Source: CAD feature listing. Evaluate the final solid. Frame: model axes, mm. A direction names the side the tool comes from. Give positions to 0.01 mm unless a question says otherwise; leave off trailing zeros. Write each loop counter-clockwise with the first axis right and the second up, starting at its lowest first coordinate (ties: lowest second). Pieces come first, ordered by that corner, then holes.
```python
from build123d import *

# Parameters (mm, degrees)
SKETCH_1_R          = 2
EXTRUDE_1_DEPTH     = 4
FILLET_1_R          = 10
FILLET_2_R          = 2
SKETCH_8_R          = 3.300000000000001
EXTRUDE_3_DEPTH     = 5
CHAMFER_1_SIZE      = 5
SKETCH_9_R          = 3.300000000000001
CUT_EXTRUDE_3_DEPTH = 5
CHAMFER_2_SIZE      = 5
SKETCH_10_R         = 5.5
SKETCH_10_R_2       = 3.3000000000000003
EXTRUDE_4_DEPTH     = 4
SKETCH_11_R         = 3.3000000000000007
CUT_EXTRUDE_4_DEPTH = 4
FILLET_3_R          = 5
SKETCH_12_R         = 1.7999999999999998
SKETCH_12_R_2       = 1.800000000000001
SKETCH_12_R_3       = 1.7999999999999972
SKETCH_12_R_4       = 1.8000000000000007
CUT_EXTRUDE_5_DEPTH = 10


with BuildPart() as part:
    # ｽｹｯﾁ1 → ﾎﾞｽ - 押し出し1 (new body)
    # profile 1 of 5: a face of its own
    with BuildSketch(Plane.XY):
        with BuildLine():
            ThreePointArc((-27.5, 2.1540659228538024), (-27.33345237791561, 2.333452377915602), (-27.15406592285381, 2.49999999999999))
            Line((-27.154065922853814, 2.499999999999997), (-27.499999999999996, 2.499999999999997))
            Line((-27.499999999999996, 2.499999999999997), (-27.499999999999996, 2.154065922853802))
        make_face()
    # profile 2 of 5: a face of its own
    with BuildSketch(Plane.XY):
        with BuildLine():
            Line((-27.5, -2.500000000000003), (-27.154065922853817, -2.500000000000003))
            ThreePointArc((-27.154065922853817, -2.499999999999992), (-27.333452377915613, -2.3334523779156044), (-27.5, -2.1540659228538055))
            Line((-27.5, -2.1540659228538055), (-27.5, -2.500000000000003))
        make_face()
    # profile 3 of 5: a face of its own
    with BuildSketch(Plane.XY):
        with BuildLine():
            ThreePointArc((-20.10102051443362, 2.49999999999994), (-30.499999999999996, -2.39e-15), (-20.101020514433618, -2.4999999999999454))
            Line((-20.1010205144336, -2.500000000000002), (-22.84593407714621, -2.5000000000000027))
            ThreePointArc((-22.845934077146207, -2.5000000000000133), (-25.000000000000018, -3.3000000000000043), (-27.154065922853817, -2.499999999999992))
            Line((-27.154065922853817, -2.500000000000003), (-27.5, -2.500000000000003))
            Line((-27.5, -2.500000000000003), (-27.5, -2.1540659228538055))
            ThreePointArc((-27.5, -2.1540659228538055), (-28.3, -1.19e-15), (-27.5, 2.1540659228538024))
            Line((-27.499999999999996, 2.154065922853802), (-27.499999999999996, 2.499999999999997))
            Line((-27.499999999999996, 2.499999999999997), (-27.154065922853814, 2.499999999999997))
            ThreePointArc((-27.15406592285381, 2.49999999999999), (-25.000000000000014, 3.299999999999998), (-22.845934077146207, 2.500000000000007))
            Line((-22.84593407714621, 2.4999999999999982), (-20.1010205144336, 2.4999999999999987))
        make_face()
    # profile 4 of 5: a face of its own
    with BuildSketch(Plane.XY):
        with BuildLine():
            Line((-22.84593407714621, -2.5000000000000027), (-20.1010205144336, -2.500000000000002))
            ThreePointArc((-20.101020514433618, -2.4999999999999454), (-19.652365608485606, -1.2856151891963796), (-19.500000000000004, -4.41e-15))
            ThreePointArc((-19.500000000000004, -3.06e-15), (-19.652365608485606, 1.2856151891963756), (-20.10102051443362, 2.49999999999994))
            Line((-20.1010205144336, 2.4999999999999987), (-22.84593407714621, 2.4999999999999982))
            ThreePointArc((-22.845934077146207, 2.5000000000000067), (-22.00013187411367, 1.3750604449591433), (-21.7, -3.06e-15))
            ThreePointArc((-21.7, -3.87e-15), (-22.00013187411367, -1.3750604449591517), (-22.845934077146207, -2.5000000000000133))
        make_face()
    # profile 5 of 5: a face of its own
    with BuildSketch(Plane.XY):
        with BuildLine():
            Line((-20.1010205144336, -2.500000000000002), (2.5, -2.4999999999999996))
            Line((2.5, -2.4999999999999996), (2.499999999999999, 2.500000000000005))
            Line((2.499999999999999, 2.500000000000005), (-20.1010205144336, 2.4999999999999987))
            ThreePointArc((-20.10102051443362, 2.49999999999994), (-19.652365608485606, 1.2856151891963756), (-19.500000000000004, -3.06e-15))
            ThreePointArc((-19.500000000000004, -4.41e-15), (-19.652365608485606, -1.2856151891963796), (-20.101020514433618, -2.4999999999999454))
        make_face()
        Circle(SKETCH_1_R, mode=Mode.SUBTRACT)
    extrude(amount=EXTRUDE_1_DEPTH)

    # ﾌｨﾚｯﾄ1
    fillet_1_edges = [part.edges().sort_by_distance(p)[0] for p in [
        (-20.10102051443361, 2.4999999999999694, 2),
        (-20.10102051443361, -2.4999999999999742, 2),
    ]]
    fillet(fillet_1_edges, radius=FILLET_1_R)

    # ﾌｨﾚｯﾄ2
    fillet_2_edges = [part.edges().sort_by_distance(p)[0] for p in [
        (2.499999999999999, 2.500000000000005, 2),
        (2.5, -2.4999999999999996, 2),
    ]]
    fillet(fillet_2_edges, radius=FILLET_2_R)

    # ｽｹｯﾁ8 → ﾎﾞｽ - 押し出し3 (add)
    with BuildSketch(Plane(origin=(0, 0, 0), x_dir=(-1, 0, 0), z_dir=(0, 0, -1))):
        with BuildLine():
            Line((15.83484861008833, 2.5), (15.834848610088294, -2.500000000000004))
            ThreePointArc((15.834848610088294, -2.500000000000004), (18.945703694279587, -2.996180733770167), (21.747849506805537, -4.435483870967743))
            ThreePointArc((21.747849506805537, -4.435483870967743), (30.499999999999996, -3.06e-15), (21.747849506805537, 4.435483870967737))
            ThreePointArc((21.747849506805537, 4.435483870967737), (18.9457036942796, 2.996180733770169), (15.83484861008833, 2.5))
        make_face()
        with Locations((25, -3.06e-15)):
            Circle(SKETCH_8_R, mode=Mode.SUBTRACT)
    extrude(amount=EXTRUDE_3_DEPTH)

    # 面取り1
    chamfer_1_edges = [part.edges().sort_by_distance(p)[0] for p in [
        (-15.834848610088311, -1.78e-15, 0),
    ]]
    chamfer(chamfer_1_edges, length=CHAMFER_1_SIZE - 0.0001)  # a hair under: the kernel refuses the full size

    # ｽｹｯﾁ9 → ｶｯﾄ - 押し出し3 (cut)
    with BuildSketch(Plane.XY.offset(4)):
        with BuildLine():
            Line((-18.834848610088333, -2.960607985830548), (-18.83484861008833, 2.9606079858305425))
            ThreePointArc((-18.83484861008833, 2.9606079858305425), (-20.351950663989726, 3.5783527846792875), (-21.747849506805537, 4.435483870967737))
            ThreePointArc((-21.747849506805537, 4.435483870967737), (-30.499999999999996, -1.29e-15), (-21.747849506805537, -4.435483870967743))
            ThreePointArc((-21.747849506805537, -4.435483870967743), (-20.35195066398973, -3.5783527846792946), (-18.834848610088333, -2.960607985830548))
        make_face()
        with Locations(Location((-25, -3.06e-15, 0), (0, 0, 180))):
            Circle(SKETCH_9_R, mode=Mode.SUBTRACT)
    extrude(amount=-CUT_EXTRUDE_3_DEPTH, mode=Mode.SUBTRACT)

    # 面取り2
    chamfer_2_edges = [part.edges().sort_by_distance(p)[0] for p in [
        (-18.83484861008833, -2.66e-15, 4),
    ]]
    chamfer(chamfer_2_edges, length=CHAMFER_2_SIZE - 0.0001)  # a hair under: the kernel refuses the full size

    # ｽｹｯﾁ10 → ﾎﾞｽ - 押し出し4 (add)
    with BuildSketch(Plane(origin=(0, 0, 0), x_dir=(-1, 0, 0), z_dir=(0, 0, -1))):
        Circle(SKETCH_10_R)
        Circle(SKETCH_10_R_2, mode=Mode.SUBTRACT)
    extrude(amount=-EXTRUDE_4_DEPTH)

    # ｽｹｯﾁ11 → ｶｯﾄ - 押し出し4 (cut)
    with BuildSketch(Plane(origin=(0, 0, 0), x_dir=(-1, 0, 0), z_dir=(0, 0, -1))):
        Circle(SKETCH_11_R)
    extrude(amount=-CUT_EXTRUDE_4_DEPTH, mode=Mode.SUBTRACT)

    # ﾌｨﾚｯﾄ3
    fillet_3_edges = [part.edges().sort_by_distance(p)[0] for p in [
        (-4.898979485566355, 2.5000000000000027, 2),
        (-4.898979485566356, -2.5000000000000004, 2),
    ]]
    fillet(fillet_3_edges, radius=FILLET_3_R)

    # ｽｹｯﾁ12 → ｶｯﾄ - 押し出し5 (cut)
    with BuildSketch(Plane.XY.offset(4)):
        with Locations((-6.8141053858085305, -1.6024880002863613)):
            Circle(SKETCH_12_R)
        with Locations((-0.8630886568357895, -6.946587505419047)):
            Circle(SKETCH_12_R_2)
        with Locations((6.814105385815693, 1.6024880002767492)):
            Circle(SKETCH_12_R_3)
        with Locations((0.8630886568356403, 6.946587505418688)):
            Circle(SKETCH_12_R_4)
    extrude(amount=-CUT_EXTRUDE_5_DEPTH, mode=Mode.SUBTRACT)


solid = part.part
```
1. Section query A-A (y = -1.75). Give the number of separate pieces and of enclosed holes in the cut face, plus the area to 3 significant figures.
2. Pull-direction query (X, two-part tool) for faces 4 (the flat face through (-13, -2.5, 0)), 5 (the flat face through (-13.3, 0.035, -2.465)), 6 (the cylindrical face through (-28.15, 0.99, -2.97)), 7 (the flat face through (-4, 0, 4)); classes: pulls with the +X half, pulls with the -X half, needs draft (parallel to the pull), parting line crosses it, or undercut.
3. Section query C-C (z = 2.5). Return loops of the section in (x, y).
4. Section query B-B (x = -25). Return loops of the section in (y, z).
5. Line query: probe 1 along X at (y, z) = (-0.75, 3.25); probe 2 along X at (y, z) = (-2.25, 1); probe 3 along Y at (x, z) = (-25, -3.95). Output: solid intervals per line, ascending.
6. Pin query (flat end, axial travel): P1, Ø1, axis at x = -1, z = -1.5, coming from the -Y side; P2, Ø2, axis at x = -14, y = 0.5, coming from the -Z side; P3, Ø4, axis at x = -16.5, z = 2, coming from the +Y side; P4, Ø4.5, axis at x = -6.81, y = -1.6, coming from the -Z side. Return the tip coordinate at first contact, or that it passes through.
7. Access query for faces 1 (the flat face through (-3, -2, 0)), 2 (the flat face through (-22, -2, -1)), 3 (the flat face through (-21, 0, -5)). Directions: +Z, -Z, +X, -X, +Y, -Y. A direction counts if a zero-diameter tool reaches every point of the face in a straight line with its end or side. Return the directions, or none.
8. Section query D-D (z = 0.75). Return loops of the section in (x, y), plus the area to 3 significant figures.
The answers:
1. separate pieces: 4
1. enclosed holes: 0
1. area: 97.6 mm2
2. face 4: undercut
2. face 5: pulls with the +X half
2. face 6: undercut
2. face 7: needs draft
3. outline: (-15.33, -2.5) - (-8.37, -2.5) arc R1.8 cw (long way) to (-5.51, -2.85) arc R5 cw to (-3.85, -3.93) arc R5.5 ccw to (-1.54, -5.28) arc R1.8 cw to (0.2, -5.5) arc R5.5 ccw to (5.49, 0.39) arc R1.8 cw to (5.08, 2.1) arc R5.5 ccw to (1.54, 5.28) arc R1.8 cw to (-0.2, 5.5) arc R5.5 ccw to (-3.85, 3.93) arc R5 cw to (-7.35, 2.5) - (-15.33, 2.5) - close; hole circle Ø6.6 at (0, 0)
4. outline: (-5.5, -5) - (-3.3, -5) - (-3.3, -1) - (-5.5, -1) - close; (3.3, -5) - (5.5, -5) - (5.5, -1) - (3.3, -1) - close
5. probe 1: x = -14.58 to -8.4, -5.23 to -3.21, 3.21 to 5.45
5. probe 2: x = -16.83 to -8.49, -5.13 to -2.41, 2.41 to 5.02
5. probe 3: y = -5.5 to -3.3, 3.3 to 5.5
6. P1: passes through
6. P2: stops at z = -4.17
6. P3: stops at y = 2.65
6. P4: stops at z = 0
7. face 1: -Z, +X, +Y, -Y
7. face 2: +Z, -X, +Y, -Y
7. face 3: -Z, +X, -X, +Y, -Y
8. outline: (-17.08, -2.58) arc R10 cw to (-15.83, -2.5) - (-8.37, -2.5) arc R1.8 cw (long way) to (-5.51, -2.85) arc R5 cw to (-3.85, -3.93) arc R5.5 ccw to (-1.54, -5.28) arc R1.8 cw to (0.2, -5.5) arc R5.5 ccw to (5.49, 0.39) arc R1.8 cw to (5.08, 2.1) arc R5.5 ccw to (1.54, 5.28) arc R1.8 cw to (-0.2, 5.5) arc R5.5 ccw to (-3.85, 3.93) arc R5 cw to (-7.35, 2.5) - (-15.83, 2.5) arc R10 cw to (-17.08, 2.58) - close; hole circle Ø6.6 at (0, 0)
8. area: 112 mm2
